from build123d import *

# Parameters (mm, degrees)
SKETCH_1_W          = 1070
SKETCH_1_H          = 1530
EXTRUDE_1_DEPTH     = 15
SKETCH_2_R          = 40
SKETCH_2_R_2        = 60
SKETCH_2_R_3        = 10
CUT_EXTRUDE_1_DEPTH = 934.996788003
CUT_EXTRUDE_2_DEPTH = 15
SKETCH_5_R          = 3
CUT_EXTRUDE_3_DEPTH = 934.996788003


with BuildPart() as part:
    # Эскиз1 → Бобышка-Вытянуть1 (new, symmetric)
    with BuildSketch(Plane.XY):
        Rectangle(SKETCH_1_W, SKETCH_1_H)
    extrude(amount=EXTRUDE_1_DEPTH, both=True)

    # Эскиз2 → Вырез-Вытянуть1 (cut, through all)
    with BuildSketch(Plane.XY.offset(15)):
        with Locations((215, -225)):
            Circle(SKETCH_2_R)
        with Locations((225, -465)):
            Circle(SKETCH_2_R_2)
        with Locations((25, -465)):
            Circle(SKETCH_2_R_2)
        with Locations((210, 360)):
            Circle(SKETCH_2_R_3)
        with Locations((-210, -350)):
            Circle(SKETCH_2_R_3)
        with BuildLine():
            Line((-30, 325), (70, 325))
            ThreePointArc((70, 325), (105.355339059, 310.355339059), (120, 275))
            Line((120, 275), (120, 100))
            ThreePointArc((120, 100), (105.355339059, 64.644660941), (70, 50))
            Line((70, 50), (-30, 50))
            ThreePointArc((-30, 50), (-65.355339059, 64.644660941), (-80, 100))
            Line((-80, 100), (-80, 275))
            ThreePointArc((-80, 275), (-65.355339059, 310.355339059), (-30, 325))
        make_face()
    extrude(amount=-CUT_EXTRUDE_1_DEPTH, mode=Mode.SUBTRACT)

    # Эскиз4 → Вырез-Вытянуть2 (cut)
    with BuildSketch(Plane.XY.offset(15)):
        with BuildLine():
            Line((495, -105), (525, -105))
            ThreePointArc((525, -105), (532.071067812, -107.928932188), (535, -115))
            Line((535, -115), (535, -165))
            ThreePointArc((535, -165), (532.071067812, -172.071067812), (525, -175))
            Line((525, -175), (495, -175))
            ThreePointArc((495, -175), (487.928932188, -172.071067812), (485, -165))
            Line((485, -165), (485, -115))
            ThreePointArc((485, -115), (487.928932188, -107.928932188), (495, -105))
        make_face()
        with BuildLine():
            Line((495, -630), (525, -630))
            ThreePointArc((525, -630), (532.071067812, -632.928932188), (535, -640))
            Line((535, -640), (535, -690))
            ThreePointArc((535, -690), (532.071067812, -697.071067812), (525, -700))
            Line((525, -700), (495, -700))
            ThreePointArc((495, -700), (487.928932188, -697.071067812), (485, -690))
            Line((485, -690), (485, -640))
            ThreePointArc((485, -640), (487.928932188, -632.928932188), (495, -630))
        make_face()
        with BuildLine():
            Line((-410, -615), (-360, -615))
            ThreePointArc((-360, -615), (-352.928932188, -617.928932188), (-350, -625))
            Line((-350, -625), (-350, -755))
            ThreePointArc((-350, -755), (-352.928932188, -762.071067812), (-360, -765))
            Line((-360, -765), (-410, -765))
            ThreePointArc((-410, -765), (-417.071067812, -762.071067812), (-420, -755))
            Line((-420, -755), (-420, -625))
            ThreePointArc((-420, -625), (-417.071067812, -617.928932188), (-410, -615))
        make_face()
        with BuildLine():
            Line((495, 725), (525, 725))
            ThreePointArc((525, 725), (532.071067812, 722.071067812), (535, 715))
            Line((535, 715), (535, 665))
            ThreePointArc((535, 665), (532.071067812, 657.928932188), (525, 655))
            Line((525, 655), (495, 655))
            ThreePointArc((495, 655), (487.928932188, 657.928932188), (485, 665))
            Line((485, 665), (485, 715))
            ThreePointArc((485, 715), (487.928932188, 722.071067812), (495, 725))
        make_face()
        with BuildLine():
            Line((335, -615), (385, -615))
            ThreePointArc((385, -615), (392.071067812, -617.928932188), (395, -625))
            Line((395, -625), (395, -755))
            ThreePointArc((395, -755), (392.071067812, -762.071067812), (385, -765))
            Line((385, -765), (335, -765))
            ThreePointArc((335, -765), (327.928932188, -762.071067812), (325, -755))
            Line((325, -755), (325, -625))
            ThreePointArc((325, -625), (327.928932188, -617.928932188), (335, -615))
        make_face()
    extrude(amount=-CUT_EXTRUDE_2_DEPTH, mode=Mode.SUBTRACT)

    # Эскиз5 → Вырез-Вытянуть3 (cut, through all)
    with BuildSketch(Plane.XY.offset(15)):
        with Locations((-475, 690)):
            Circle(SKETCH_5_R)
        with Locations((-5, 690)):
            Circle(SKETCH_5_R)
        with Locations((425, 690)):
            Circle(SKETCH_5_R)
        with Locations((-475, -135)):
            Circle(SKETCH_5_R)
        with Locations((-5, -215)):
            Circle(SKETCH_5_R)
        with Locations((425, -215)):
            Circle(SKETCH_5_R)
        with Locations((-465, -675)):
            Circle(SKETCH_5_R)
        with Locations((10, -675)):
            Circle(SKETCH_5_R)
        with Locations((435, -675)):
            Circle(SKETCH_5_R)
    extrude(amount=-CUT_EXTRUDE_3_DEPTH, mode=Mode.SUBTRACT)


solid = part.part
For this review, take the finished solid that the model builds, in its own axes (mm). A direction names the side the tool comes from. Give positions to 0.01 mm unless a question says otherwise; leave off trailing zeros. Write each loop counter-clockwise with the first axis right and the second up, starting at its lowest first coordinate (ties: lowest second). Pieces come first, ordered by that corner, then holes. Notation, with made-up numbers: (80, 50.5) -> (125, 50.5) arc R17 ccw to (125, 76.5) -> close; hole circle Ø3 at (43, 68). An arc over 180 degrees is marked (long way). Use CSV: the item, a comma, the result in double quotes.
Q1. Take a section at B-B, the plane z = 6. State how many separate pieces and enclosed holes the cut face has, then the cut area to 3 significant figures.
Conclusion:
separate pieces,"1"
enclosed holes,"15"
area,"1,520,000 mm2"
Q2. Take a section at A-A, the plane y = 198.5. Write out the cut boundary in (x, z), then the cut area to 3 significant figures.
Conclusion:
outline,"(-535, -15) -> (-80, -15) -> (-80, 15) -> (-535, 15) -> close; (120, -15) -> (535, -15) -> (535, 15) -> (120, 15) -> close"
area,"26,100 mm2"
Q3. For P1, Ø8, axis at x = -5, y = -215, coming from the -Z side; P2, Ø12, axis at y = -652.5, z = 8, coming from the +X side; P3, Ø5, axis at x = 435, y = -675, coming from the -Z side, all flat-tipped, find the tip position at first contact; note any pin that passes through.
Conclusion:
P1,"z = -15"
P2,"x = 485"
P3,"through"
Q4. To check wall thickness, follow probe 1 along X at (y, z) = (-675, -5.25); probe 2 along X at (y, z) = (690, 3.75); probe 3 along Y at (x, z) = (25, 5). State the ranges of each line that lie inside material, in increasing order. Write a range as [from, to].
Conclusion:
probe 1,"[-535, -468], [-462, 7], [13, 432], [438, 535]"
probe 2,"[-535, -478], [-472, -8], [-2, 422], [428, 485]"
probe 3,"[-765, -525], [-405, 50], [325, 765]"
Q5. Tool access review of faces 4 (the face through (510, -140, 0)), 5 (the face through (-535, -11, 0)), 6 (the face through (-65.742, 309.964, 0.21)): name each direction out of +Z, -Z, +X, -X, +Y, -Y from which nothing blocks a thin tool from reaching the whole face with its end or side.
Conclusion:
face 4,"+Z"
face 5,"+Z, -Z, -X, +Y, -Y"
face 6,"+Z, -Z"
Q6. Mouldability with a two-part tool opening along Y and no side actions: class faces 1 (the face through (535, -11, 0)), 2 (the face through (-7, 765, 0)), 3 (the face through (-385, -689, 0)) as pulls with the +Y half, pulls with the -Y half, needs draft (parallel to the pull), parting line crosses it, or undercut.
Conclusion:
face 1,"needs draft"
face 2,"pulls with the +Y half"
face 3,"undercut"
